```python
from build123d import *

# Parameters (mm, degrees)
F0_W      = 101.6
F0_H      = 32.004
F1_DEPTH  = 6.35
F2_R      = 2.372595
F3_DEPTH  = 3.048
F4_R      = 0.508
F5_W      = 16.002
F5_H      = 29.0068
F5_R      = 3.2512
F5_R_2    = 2.4003
F6_DEPTH  = 3.5052
F7_W      = 101.6
F7_H      = 3.175
F8_DEPTH  = 6.35
F9_W      = 38.1
F9_H      = 7.62
F10_DEPTH = 6.35


with BuildPart() as f1:
    # F0 (on Top) → F1 (new body)
    with BuildSketch(Plane.XY):
        with Locations((50.8, 16.002)):
            Rectangle(F0_W, F0_H)
    extrude(amount=F1_DEPTH)

    # F2 (on face) → F3 (join)
    with BuildSketch(Plane.XY.offset(6.35)):
        with Locations((12.0015, 20.0025)):
            Circle(F2_R)
        with Locations((12.0015, 12.0015)):
            Circle(F2_R)
        with BuildLine():
            ThreePointArc((6.373095, 12.0015), (5.678178, 13.679178), (4.0005, 14.374095))
            ThreePointArc((4.0005, 14.374095), (2.322822, 10.323822), (6.373095, 12.0015))
        make_face()
        with BuildLine():
            ThreePointArc((4.0005, 17.629905), (5.678178, 18.324822), (6.373095, 20.0025))
            ThreePointArc((6.373095, 20.0025), (2.322822, 21.680178), (4.0005, 17.629905))
        make_face()
    extrude(amount=F3_DEPTH)

    # F4
    f4_edges = [f1.edges().sort_by_distance(p)[0] for p in [
        (9.628905, 20.0025, 9.398),
        (4.0005, 22.375095, 9.398),
        (1.627905, 12.0015, 9.398),
        (9.628905, 12.0015, 9.398),
    ]]
    fillet(f4_edges, radius=F4_R)

    # F5 (on face) → F6 (cut)
    with BuildSketch(Plane(origin=(0, 0, 0), x_dir=(1, 0, 0), z_dir=(0, 0, -1))):
        with Locations((8.89, -16.002)):
            Rectangle(F5_W, F5_H)
        with Locations((8.89, -24.003)):
            Circle(F5_R, mode=Mode.SUBTRACT)
        with Locations((8.89, -16.002)):
            Circle(F5_R, mode=Mode.SUBTRACT)
        with Locations((8.89, -8.001)):
            Circle(F5_R, mode=Mode.SUBTRACT)
        with Locations((92.71, -16.002)):
            Rectangle(F5_W, F5_H)
        with Locations((92.71, -24.003)):
            Circle(F5_R, mode=Mode.SUBTRACT)
        with Locations((92.71, -16.002)):
            Circle(F5_R, mode=Mode.SUBTRACT)
        with Locations((92.71, -8.001)):
            Circle(F5_R, mode=Mode.SUBTRACT)
        with Locations((8.89, -8.001)):
            Circle(F5_R_2)
        with Locations((8.89, -16.002)):
            Circle(F5_R_2)
        with Locations((8.89, -24.003)):
            Circle(F5_R_2)
        with Locations((92.71, -8.001)):
            Circle(F5_R_2)
        with Locations((92.71, -16.002)):
            Circle(F5_R_2)
        with Locations((92.71, -24.003)):
            Circle(F5_R_2)
    extrude(amount=-F6_DEPTH, mode=Mode.SUBTRACT)

    # F7 (on face) → F8 (cut, through all)
    with BuildSketch(Plane(origin=(0, 0, 0), x_dir=(1, 0, 0), z_dir=(0, 0, -1))):
        with Locations((50.8, -30.4165)):
            Rectangle(F7_W, F7_H)
        with Locations((50.8, -1.5875)):
            Rectangle(F7_W, F7_H)
    extrude(amount=-F8_DEPTH, mode=Mode.SUBTRACT)

    # F9 (on face) → F10 (cut, through all)
    with BuildSketch(Plane.XY.offset(6.35)):
        with Locations((50.8, 16.002)):
            Rectangle(F9_W, F9_H)
    extrude(amount=-F10_DEPTH, mode=Mode.SUBTRACT)


solid = f1.part
```
Here's how the part is built. I have some questions about the finished solid (model axes, mm). A direction names the side the tool comes from. Coordinates: 2 decimals unless noted, no trailing zeros. Write each loop counter-clockwise with the first axis right and the second up, starting at its lowest first coordinate (ties: lowest second). Pieces come first, ordered by that corner, then holes. Notation, with made-up numbers: (82, 80.5) -> (99, 80.5) arc R13 ccw to (99, 91.5) -> close; hole circle Ø6 at (77.5, 81.25). An arc over 180 degrees is marked (long way). Use a Markdown table: item, result. Add a question column.
(1) If we section it at C-C, the plane x = 92.71: Write out the boundary of the cut face in (y, z) (3 decimals), and give its area (3 significant figures).
(2) If we section it at D-D, the plane x = 27.5: Write out the boundary of the cut face in (y, z) (3 decimals), and give its area (3 significant figures).
(3) If we section it at B-B, the plane x = 65.5: Write out the boundary of the cut face in (y, z) (3 decimals).
(4) We'd pull the mould along X, two halves only. Please class faces 6 (the flat face through (7, 6, 0)), 7 (the flat face through (0, 16, 3)), 8 (the flat face through (51, 12.192, 3)): +X half, -X half, draft (parallel to the pull), parting line (faces both ways), or undercut.
(5) Please list where these lines run through material, in increasing order: line 1 (Y direction, x = 8.89, z = 0.85); line 2 (X direction, y = 19.75, z = 8.5); line 3 (X direction, y = 19.75, z = 5.75).
(6) If we section it at A-A, the plane z = 8: Write out the boundary of the cut face in (x, y), and give its area (3 significant figures).
(7) I'm going to push flat-ended pins straight in: P1, Ø1.4, axis at x = 93, y = 25, coming from the -Z side; P2, Ø1, axis at x = 30.5, y = 12.5, coming from the +Z side. Where does each tip first touch, or does it pass through?
(8) For faces 1 (the flat face through (69.85, 16, 3)), 2 (the flat face through (12, 12, 9.398)), 3 (the cylindrical face through (10.12, 18.56, 7.6)), 4 (the flat face through (100.711, 16, 2)), 5 (the flat face through (9, 16, 3.505)), which set-ups out of +Z, -Z, +X, -X, +Y, -Y let a thin tool reach every point of the face, with its end or its side?
Outcome:
| question | item | result |
|---|---|---|
| 1 | outline | (3.175, 3.505) -> (4.75, 3.505) -> (4.75, 0) -> (5.601, 0) -> (5.601, 3.505) -> (10.401, 3.505) -> (10.401, 0) -> (11.252, 0) -> (11.252, 3.505) -> (12.751, 3.505) -> (12.751, 0) -> (13.602, 0) -> (13.602, 3.505) -> (18.402, 3.505) -> (18.402, 0) -> (19.253, 0) -> (19.253, 3.505) -> (20.752, 3.505) -> (20.752, 0) -> (21.603, 0) -> (21.603, 3.505) -> (26.403, 3.505) -> (26.403, 0) -> (27.254, 0) -> (27.254, 3.505) -> (28.829, 3.505) -> (28.829, 6.35) -> (3.175, 6.35) -> close |
| 1 | area | 90.9 mm^2 |
| 2 | outline | (3.175, 0) -> (28.829, 0) -> (28.829, 6.35) -> (3.175, 6.35) -> close |
| 2 | area | 163 mm^2 |
| 3 | outline | (3.175, 0) -> (12.192, 0) -> (12.192, 6.35) -> (3.175, 6.35) -> close; (19.812, 0) -> (28.829, 0) -> (28.829, 6.35) -> (19.812, 6.35) -> close |
| 4 | face 6 | draft |
| 4 | face 7 | -X half |
| 4 | face 8 | undercut |
| 5 | line 1 | y = 4.75 to 5.6, 10.4 to 11.25, 12.75 to 13.6, 18.4 to 19.25, 20.75 to 21.6, 26.4 to 27.25 |
| 5 | line 2 | x = 1.64 to 6.36, 9.64 to 14.36 |
| 5 | line 3 | x = 0 to 31.75, 69.85 to 101.6 |
| 6 | outline | circle Ø4.75 at (4, 12); circle Ø4.75 at (4, 20); circle Ø4.75 at (12, 12); circle Ø4.75 at (12, 20) |
| 6 | area | 70.7 mm^2 |
| 7 | P1 | stops at z = 3.51 |
| 7 | P2 | stops at z = 6.35 |
| 8 | face 1 | +Z, -Z |
| 8 | face 2 | +Z, +X, -X, +Y, -Y |
| 8 | face 3 | +Z |
| 8 | face 4 | -Z, +Y, -Y |
| 8 | face 5 | -Z |
